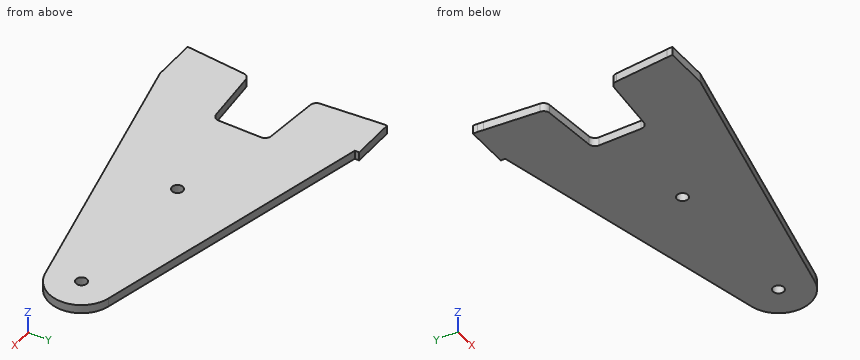
from build123d import *

# Parameters (mm, degrees)
SKETCH1_R           = 2.55
BOSS_EXTRUDE1_DEPTH = 4


with BuildPart() as part:
    # Sketch1 → Boss-Extrude1 (new body)
    with BuildSketch(Plane.XY):
        with BuildLine():
            Line((14.872885109, 17.599965411), (12.706250758, 42.361500851))
            Line((12.706250758, 42.361500851), (12.474619372, 45.008716695))
            Line((12.474619372, 45.008716695), (12.474619372, 47))
            Line((12.474619372, 47), (32.474619372, 47))
            Line((32.474619372, 47), (32.474619372, 45))
            Line((32.474619372, 45), (162.509181482, 14.606317485))
            ThreePointArc((162.509181482, 14.606317485), (174.095167783, 0), (162.509181482, -14.606317485))
            Line((162.509181482, -14.606317485), (32.474619372, -45))
            Line((32.474619372, -45), (12.474619372, -45.008716695))
            Line((12.474619372, -45.008716695), (12.706250758, -42.361500851))
            Line((12.706250758, -42.361500851), (14.872885109, -17.599965411))
            ThreePointArc((14.872885109, -17.599965411), (15.740145918, -15.740145918), (17.599965411, -14.872885109))
            Line((17.599965411, -14.872885109), (42.361500851, -12.706250758))
            ThreePointArc((42.361500851, -12.706250758), (44.311843411, -11.744427787), (45.1, -9.717669606))
            Line((45.1, -9.717669606), (45.1, 9.717669606))
            ThreePointArc((45.1, 9.717669606), (44.311843411, 11.744427787), (42.361500851, 12.706250758))
            Line((42.361500851, 12.706250758), (17.599965411, 14.872885109))
            ThreePointArc((17.599965411, 14.872885109), (15.740145918, 15.740145918), (14.872885109, 17.599965411))
        make_face()
        with Locations((159.095167783, 0)):
            Circle(SKETCH1_R, mode=Mode.SUBTRACT)
        with Locations((90, 0)):
            Circle(SKETCH1_R, mode=Mode.SUBTRACT)
    extrude(amount=BOSS_EXTRUDE1_DEPTH)


solid = part.part
Read the model definition and answer for the solid it produces. Units are mm, in the model's axes. Coordinates: 2 decimals unless noted, no trailing zeros. Loops run counter-clockwise (first coordinate to the right, second up) from the corner with the lowest first, then second, coordinate; pieces in that order, holes last. Notation, with made-up numbers: (-8, -0.5) - (40, -0.5) arc R18 cw to (40, 8.5) - close; hole circle Ø5 at (18.5, 33.5). An arc over 180 degrees is marked (long way). Answer in a Markdown table with one row per item.
Q1. Given P1, Ø1.6, axis at y = 46.5, z = 1.5, coming from the +X side; P2, Ø1.5, axis at x = 76.5, z = 2.5, coming from the -Y side (3 decimals); P3, Ø8, axis at x = 102, y = 33.5, coming from the -Z side; P4, Ø2, axis at y = 20.5, z = 1.5, coming from the -X side, each flat-ended and moving along its own axis, determine where each tip first touches the part or whether it passes through.
Here are the results:
| item | result |
|---|---|
| P1 | stops at x = 32.47 |
| P2 | stops at y = -34.885 |
| P3 | passes through |
| P4 | stops at x = 14.53 |
Q2. Find section B-B on z = 1.15. Write down the section's boundary in (x, y).
Here are the results:
| item | result |
|---|---|
| outline | (12.47, -45.01) - (32.47, -45) - (162.51, -14.61) arc R15 ccw to (162.51, 14.61) - (32.47, 45) - (32.47, 47) - (12.47, 47) - (12.47, 45.01) - (14.87, 17.6) arc R3 ccw to (17.6, 14.87) - (42.36, 12.71) arc R3 cw to (45.1, 9.72) - (45.1, -9.72) arc R3 cw to (42.36, -12.71) - (17.6, -14.87) arc R3 ccw to (14.87, -17.6) - close; hole circle Ø5.1 at (90, 0); hole circle Ø5.1 at (159.1, 0) |
Q3. Find section D-D on x = 134.5. Write down the section's boundary in (y, z).
Here are the results:
| item | result |
|---|---|
| outline | (-21.15, 0) - (21.15, 0) - (21.15, 4) - (-21.15, 4) - close |
Q4. Find section A-A on y = 0. Write down the section's boundary in (x, z), plus the area to 3 significant figures.
Here are the results:
| item | result |
|---|---|
| outline | (45.1, 0) - (87.45, 0) - (87.45, 4) - (45.1, 4) - close; (92.55, 0) - (156.55, 0) - (156.55, 4) - (92.55, 4) - close; (161.65, 0) - (174.1, 0) - (174.1, 4) - (161.65, 4) - close |
| area | 475 mm^2 |
Q5. Straight lines are drawn through the part: line 1 along X through (y, z) = (-2, 3); line 2 along Y through (x, z) = (90, 2.7); line 3 along Y through (x, z) = (117, 2.2). For each, find the intervals that lie inside material, in ascending order. Write a range as [from, to].
Here are the results:
| item | result |
|---|---|
| line 1 | x = [45.1, 88.42], [91.58, 157.51], [160.68, 173.96] |
| line 2 | y = [-31.55, -2.55], [2.55, 31.55] |
| line 3 | y = [-25.24, 25.24] |
Q6. Find section C-C on x = 37. Write down the section's boundary in (y, z), plus the area to 3 significant figures.
Here are the results:
| item | result |
|---|---|
| outline | (-43.94, 0) - (-13.18, 0) - (-13.18, 4) - (-43.94, 4) - close; (13.18, 0) - (43.94, 0) - (43.94, 4) - (13.18, 4) - close |
| area | 246 mm^2 |
